Can you work these out from the model? Positions are in its coordinate system, mm. Give positions to 0.01 mm unless a question says otherwise; leave off trailing zeros. Write each loop counter-clockwise with the first axis right and the second up, starting at its lowest first coordinate (ties: lowest second). Pieces come first, ordered by that corner, then holes.
Autodesk Inventor part; units mm, degrees
ref_plane "YZ Plane" through (0, 0, 0) normal (1, 0, 0) x (0, 1, 0)
ref_plane "XZ Plane" through (0, 0, 0) normal (0, 1, 0) x (-1, 0, 0)
ref_plane "XY Plane" through (0, 0, 0) normal (0, 0, 1) x (1, 0, 0)
sketch "Sketch1" plane through (0, 0, 0) normal (0, 0, 1) x (1, 0, 0)
  circle A0 centre (0, 0) radius 72.5
  dimension "d22" = 145
extrude "Plate1" add sketch "Sketch1" along normal blind 2
sketch "Sketch6" plane through (0, 0, 2) normal (0, 0, 1) x (1, 0, 0)
  circle A0 centre (65, 0) radius 3.5
  circle A1 centre (0, 0) radius 65 construction
  dimension "d37" = 130
  dimension "d36" = 7
extrude "Cut2" cut sketch "Sketch6" against normal blind 2
pattern_circular "Circular Pattern2" count 8 over 360 about axis through (0, 0, 0) along (0, 0, 1) of "Cut2"
equation "\"d38\" = Thickness"
equation "\"d2\" = Thickness"
equation "\"BendReliefWidth\" = Thickness"
equation "\"BendReliefDepth\" = 0.5 * Thickness"
equation "\"CornerReliefSize\" = 4 * Thickness"
equation "\"MinimumRemnant\" = 2 * Thickness"
equation "\"TransitionRadius\" = BendRadius"
equation "\"JacobiRadiusSize\" = BendRadius"
equation "\"GapSize\" = Thickness"
properties part number "TKS 3556 BOTTOM DS cup plug" material "Stainless Steel"
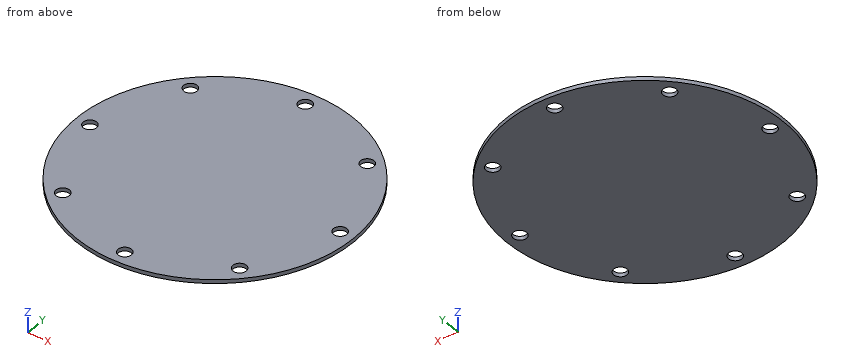
1) Please list where these lines run through material, in increasing order: L1, parallel to X at y = 1.5, z = 1.35; L2, parallel to Y at x = -2, z = 0.5; L3, parallel to Y at x = 65, z = 1.25.
Values follow:
L1: x = -72.48 to -68.16, -61.84 to 61.84, 68.16 to 72.48
L2: y = -72.47 to -67.87, -62.13 to 62.13, 67.87 to 72.47
L3: y = -32.11 to -3.5, 3.5 to 32.11
2) Suppose I cut it at A-A on y = 0. Write out the boundary of the cut face in (x, z).
Values follow:
outline: (-72.5, 0) - (-68.5, 0) - (-68.5, 2) - (-72.5, 2) - close; (-61.5, 0) - (61.5, 0) - (61.5, 2) - (-61.5, 2) - close; (68.5, 0) - (72.5, 0) - (72.5, 2) - (68.5, 2) - close
3) Suppose I cut it at B-B on x = 65. Write out the boundary of the cut face in (y, z), plus the area to 3 significant figures.
Values follow:
outline: (-32.11, 0) - (-3.5, 0) - (-3.5, 2) - (-32.11, 2) - close; (3.5, 0) - (32.11, 0) - (32.11, 2) - (3.5, 2) - close
area: 114 mm2
4) Suppose I cut it at D-D on z = 0.55. State how many separate pieces and enclosed holes the cut face has, plus the area to 3 significant figures.
Values follow:
separate pieces: 1
enclosed holes: 8
area: 16,200 mm2
5) For pin 1 Ø6.5 at (x, y) = (-65, 0) entering from -Z, with a flat end and sliding along its axis, tell me the tip position at first contact or that it passes through.
Values follow:
pin 1: passes through
